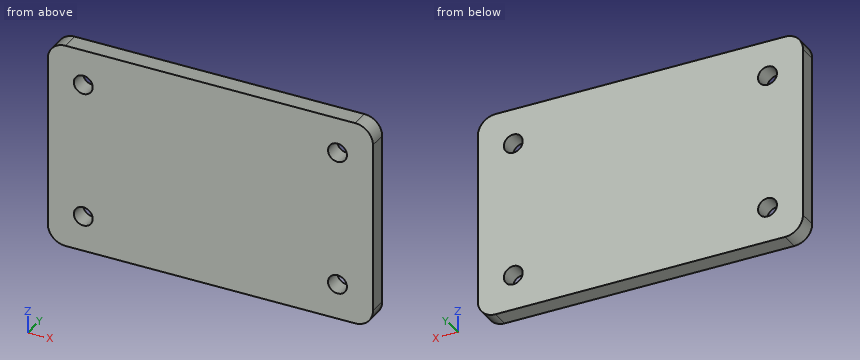
```python
from build123d import *

# Parameters (mm, degrees)
SKETCH_1_W          = 55
SKETCH_1_H          = 35
EXTRUDE_1_DEPTH     = 3
SKETCH_2_R          = 1.6
CUT_EXTRUDE_1_DEPTH = 3
FILLET_1_R          = 3


with BuildPart() as part:
    # 草图1 → 凸台-拉伸1 (new body)
    with BuildSketch(Plane(origin=(0, 0, 0), x_dir=(1, 0, 0), z_dir=(0, 1, 0))):
        with Locations((27.5, 17.5)):
            Rectangle(SKETCH_1_W, SKETCH_1_H)
    extrude(amount=EXTRUDE_1_DEPTH)

    # 草图2 → 切除-拉伸1 (cut)
    with BuildSketch(Plane(origin=(0, 3, 0), x_dir=(1, 0, 0), z_dir=(0, 1, 0))):
        with Locations(Location((6, 29, 0), (0, 0, 270))):
            Circle(SKETCH_2_R)
        with Locations(Location((49, 29, 0), (0, 0, 270))):
            Circle(SKETCH_2_R)
        with Locations(Location((49, 6, 0), (0, 0, 270))):
            Circle(SKETCH_2_R)
        with Locations(Location((6, 6, 0), (0, 0, 270))):
            Circle(SKETCH_2_R)
    extrude(amount=-CUT_EXTRUDE_1_DEPTH, mode=Mode.SUBTRACT)

    # 圆角1
    fillet_1_edges = [part.edges().sort_by_distance(p)[0] for p in [
        (0, 1.5, -35),
        (55, 1.5, -35),
        (55, 1.5, 0),
        (0, 1.5, 0),
    ]]
    fillet(fillet_1_edges, radius=FILLET_1_R)


solid = part.part
```
Part model, mm, in its own coordinate system. Give positions to 0.01 mm unless a question says otherwise; leave off trailing zeros. Write each loop counter-clockwise with the first axis right and the second up, starting at its lowest first coordinate (ties: lowest second). Pieces come first, ordered by that corner, then holes. Notation, with made-up numbers: M 28,40.5 L 43,40.5 A26 ccw 43,56.5 Z; hole C 84.5,48.5 d3. An arc over 180 degrees is marked long. Use CSV: the item, a comma, the result in double quotes.
Item 1: Slice it at A-A on z = -29. Write the cut outline in (x, y), plus the area to 3 significant figures.
Taken from the geometry:
outline,"M 0,0 L 4.4,0 L 4.4,3 L 0,3 Z; M 7.6,0 L 47.4,0 L 47.4,3 L 7.6,3 Z; M 50.6,0 L 55,0 L 55,3 L 50.6,3 Z"
area,"146 mm²"
Item 2: Drill centre lines: probe 1 along X at (y, z) = (1.3, -6); probe 2 along X at (y, z) = (1.8, -5.5); probe 3 along Z at (x, y) = (48, 0.5). Where is each one in solid material? Low to high.
Taken from the geometry:
probe 1,"x = 0 to 4.4, 7.6 to 47.4, 50.6 to 55"
probe 2,"x = 0 to 4.48, 7.52 to 47.48, 50.52 to 55"
probe 3,"z = -35 to -30.25, -27.75 to -7.25, -4.75 to 0"
Item 3: Slice it at B-B on y = 1.5. Write the cut outline in (x, z).
Taken from the geometry:
outline,"M 0,-32 A3 ccw 3,-35 L 52,-35 A3 ccw 55,-32 L 55,-3 A3 ccw 52,0 L 3,0 A3 ccw 0,-3 Z; hole C 6,-29 d3.2; hole C 6,-6 d3.2; hole C 49,-29 d3.2; hole C 49,-6 d3.2"
Item 4: Pin check, flat tip, straight feed: P1, Ø4, axis at x = 49, z = -6, coming from the -Y side. Stop position of the tip, or through.
Taken from the geometry:
P1,"stops at y = 0"
Item 5: Slice it at C-C on x = 6. Write the cut outline in (y, z).
Taken from the geometry:
outline,"M 0,-35 L 3,-35 L 3,-30.6 L 0,-30.6 Z; M 0,-27.4 L 3,-27.4 L 3,-7.6 L 0,-7.6 Z; M 0,-4.4 L 3,-4.4 L 3,0 L 0,0 Z"
